```python
from build123d import *

# Parameters (mm, degrees)
EXTRUDE_1_DEPTH          = 60
CUT_EXTRUDE_1_DEPTH      = 40
CUT_EXTRUDE_1_DEPTH_BACK = 29
SKETCH_4_R               = 15.5
SKETCH_5_W               = 5
SKETCH_5_H               = 30
CUT_EXTRUDE_2_DEPTH      = 83.900874001
SKETCH_7_W               = 60
SKETCH_7_H               = 85.424918669
EXTRUDE_2_DEPTH          = 20
CUT_EXTRUDE_START        = -31.454396
SKETCH_8_W               = 21
SKETCH_8_H               = 68.571428571
CUT_EXTRUDE_3_DEPTH      = 14


with BuildPart() as part:
    # 스케치3 → 보스-돌출1 (new body)
    with BuildSketch(Plane(origin=(0, 0, 0), x_dir=(0, 0, -1), z_dir=(1, 0, 0))):
        Polygon((-25, -51.454396413), (25, -51.454396413), (15, 4.545603587), (-15, 4.545603587), align=None)
    extrude(amount=EXTRUDE_1_DEPTH)

    # 스케치4 → 컷-돌출1 (cut, two sides: drawn at the far end of the back side and taken through both)
    with BuildSketch(Plane.XY.offset(-CUT_EXTRUDE_1_DEPTH_BACK)):
        with Locations(Location((30, -14.954396413, 0), (0, 0, 90))):
            Circle(SKETCH_4_R)
    extrude(amount=CUT_EXTRUDE_1_DEPTH + CUT_EXTRUDE_1_DEPTH_BACK, mode=Mode.SUBTRACT)

    # 스케치5 → 컷-돌출2 (cut, through all)
    with BuildSketch(Plane(origin=(0, 0, 0), x_dir=(0, 0, -1), z_dir=(1, 0, 0))):
        with Locations((0, -51.454396413)):
            Rectangle(SKETCH_5_W, SKETCH_5_H)
    extrude(amount=CUT_EXTRUDE_2_DEPTH, mode=Mode.SUBTRACT)

    # 스케치7 → 보스-돌출2 (add)
    with BuildSketch(Plane(origin=(0, -51.454396413, 0), x_dir=(-1, 0, 0), z_dir=(0, -1, 0))):
        with Locations((-30, -47.287540666)):
            Rectangle(SKETCH_7_W, SKETCH_7_H)
    extrude(amount=-EXTRUDE_2_DEPTH)

    # 스케치8 → 컷-돌출3 (cut)
    with BuildSketch(Plane(origin=(0, 0, 0), x_dir=(1, 0, 0), z_dir=(0, 1, 0)).offset(CUT_EXTRUDE_START)):
        with Locations((29.238428934, -55.714285715)):
            Rectangle(SKETCH_8_W, SKETCH_8_H)
    extrude(amount=-CUT_EXTRUDE_3_DEPTH, mode=Mode.SUBTRACT)


solid = part.part
```
Could you check a few things on this model? Use its own coordinates, in mm. A direction names the side the tool comes from. Round coordinates to 2 decimals unless told otherwise and drop trailing zeros. Write each loop counter-clockwise with the first axis right and the second up, starting at its lowest first coordinate (ties: lowest second). Pieces come first, ordered by that corner, then holes. Notation, with made-up numbers: M -3,77 L 18,77 A18 cw 18,107 Z; hole C 68,55 d5. An arc over 180 degrees is marked long. Answer in a Markdown table with one row per item. Add a question column.
Q1. Imagine slicing it at B-B (y = -2). Please give me the cut outline in (x, z), then the cut area to 3 significant figures.
Q2. If I drill on line 1 (X direction, y = -42, z = 24); line 2 (Y direction, x = 4, z = -2); line 3 (Y direction, x = 29, z = -10), over which ranges is the centre line in solid material (lowest first)? Write a range as from..to.
Q3. If we mould it in two halves opening along X, with no side actions, what happens to faces 1 (the flat face through (39.738, -38, 56)), 2 (the flat face through (0, -30, 21)), 3 (the flat face through (30, -36.454, 0))? For each: +X half, -X half, draft (parallel to the pull), parting line (faces both ways), or undercut.
Q4. Imagine slicing it at C-C (z = 67). Please give me the cut outline in (x, y).
Q5. Will these pins go through, and if not, where does the flat tip stop? pin 1 Ø6 at (x, y) = (49.5, -21) entering from +Z; pin 2 Ø11 at (x, y) = (30.5, -37.5) entering from +Z; pin 3 Ø17 at (x, z) = (30, 61) entering from +Y.
Q6. Imagine slicing it at D-D (x = 12). Please give me the cut outline in (y, z).
Q7. On a 3-axis mill with a long thin cutter (end or side, diameter ignored), from which of +Z, -Z, +X, -X, +Y, -Y can I reach the whole of each face in a straight line? I mean faces 4 (the flat face through (30, -46, 90)), 5 (the flat face through (29, -45.454, 55)), 6 (the flat face through (30, -44, -2.5)), 7 (the flat face through (50, -31.454, 55)). Say none if no direction works.
Q8. Imagine slicing it at A-A (z = 13). Please give me the cut outline in (x, y).
Values:
| question | item | result |
|---|---|---|
| 1 | outline | M 0,-16.17 L 21.49,-16.17 L 21.49,16.17 L 0,16.17 Z; M 38.51,-16.17 L 60,-16.17 L 60,16.17 L 38.51,16.17 Z |
| 1 | area | 1,390 mm^2 |
| 2 | line 1 | 0..18.74, 39.74..60 |
| 2 | line 2 | -36.45..4.55 |
| 2 | line 3 | -51.45..-30.42, 0.51..4.55 |
| 3 | face 1 | undercut |
| 3 | face 2 | -X half |
| 3 | face 3 | draft |
| 4 | outline | M 0,-51.45 L 60,-51.45 L 60,-31.45 L 39.74,-31.45 L 39.74,-45.45 L 18.74,-45.45 L 18.74,-31.45 L 0,-31.45 Z |
| 5 | pin 1 | z = 20.1 |
| 5 | pin 2 | z = 21.43 |
| 5 | pin 3 | y = -45.45 |
| 6 | outline | M -51.45,-25 L 4.55,-15 L 4.55,15 L -31.45,21.43 L -31.45,90 L -51.45,90 L -51.45,2.5 L -36.45,2.5 L -36.45,-2.5 L -51.45,-2.5 Z |
| 7 | face 4 | +Z, +X, -X, +Y, -Y |
| 7 | face 5 | +Z, +Y |
| 7 | face 6 | +X, -X, -Y |
| 7 | face 7 | +Z, +X, -X, +Y |
| 8 | outline | M 0,-51.45 L 60,-51.45 L 60,4.55 L 0,4.55 Z; hole C 30,-14.95 d31 |
